The model under review builds one solid part; all positions refer to its coordinate system, in mm. Face numbers are marked on the shaded views. A direction names the side the tool comes from. Coordinates: 2 decimals unless noted, no trailing zeros. Loops run counter-clockwise (first coordinate to the right, second up) from the corner with the lowest first, then second, coordinate; pieces in that order, holes last. Notation, with made-up numbers: M -25.5,-27.75 L 29.5,-27.75 A15 ccw 29.5,-12.75 Z; hole C 61.25,57.5 d5. An arc over 180 degrees is marked long. One line per item, written item: value.
```python
from build123d import *

# Parameters (mm, degrees)
SKETCH1_W           = 10
SKETCH1_H           = 6
BOSS_EXTRUDE1_DEPTH = 3
BOSS_EXTRUDE2_DEPTH = 6
SKETCH3_W           = 0.5
SKETCH3_H           = 2
SKETCH3_W_2         = 1
SKETCH3_H_2         = 3
CUT_EXTRUDE1_DEPTH  = 1.5


with BuildPart() as part:
    # Sketch1 → Boss-Extrude1 (new body)
    with BuildSketch(Plane.XY):
        with Locations((5, 3)):
            Rectangle(SKETCH1_W, SKETCH1_H)
    extrude(amount=BOSS_EXTRUDE1_DEPTH)

    # Sketch2 → Boss-Extrude2 (add)
    with BuildSketch(Plane.XZ):
        Polygon((3.028685262, 4.124905721), (0, 3), (5.333823351, 3), align=None)
        Polygon((7.779518642, 3.625927659), (5.333823351, 3), (10, 3), align=None)
    extrude(amount=-BOSS_EXTRUDE2_DEPTH)

    # Sketch3 → Cut-Extrude1 (cut)
    with BuildSketch(Plane(origin=(0, 0, 0), x_dir=(-1, 0, 0), z_dir=(0, 0, -1))):
        with Locations((-2.75, 3.5)):
            Rectangle(SKETCH3_W, SKETCH3_H)
        with Locations((-6.5, 3)):
            Rectangle(SKETCH3_W_2, SKETCH3_H_2)
    extrude(amount=-CUT_EXTRUDE1_DEPTH, mode=Mode.SUBTRACT)


solid = part.part
```
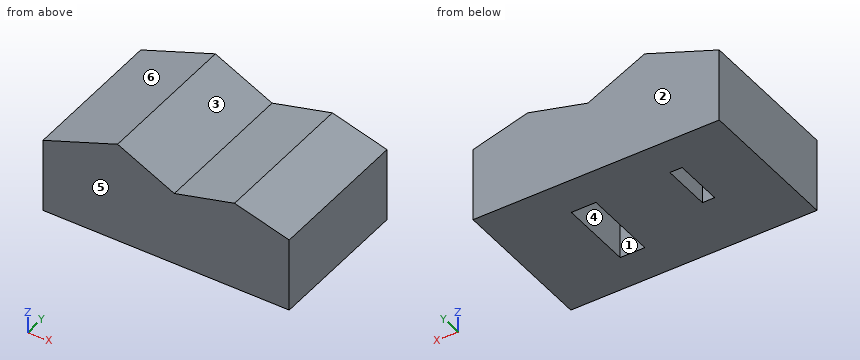
(1) Add section A-A on z = 1.15. State the section outline as (x, y) points.
Checks:
outline: M 0,0 L 10,0 L 10,6 L 0,6 Z; hole M 2.5,2.5 L 3,2.5 L 3,4.5 L 2.5,4.5 Z; hole M 6,1.5 L 7,1.5 L 7,4.5 L 6,4.5 Z
(2) Draft analysis for pull direction X (two halves, no side actions). For the marked faces 4, 5 and 6, state which applies: pulls with the +X half, pulls with the -X half, needs draft (parallel to the pull), parting line crosses it, or undercut.
Checks:
face 4: undercut
face 5: needs draft
face 6: pulls with the -X half
(3) Add section D-D on x = 6.75. State the section outline as (y, z) points, then the cut area to 3 significant figures.
Checks:
outline: M 0,0 L 1.5,0 L 1.5,1.5 L 4.5,1.5 L 4.5,0 L 6,0 L 6,3.36 L 0,3.36 Z
area: 15.7 mm^2
(4) Tool access review of the marked faces 1, 2 and 3: name each direction out of +Z, -Z, +X, -X, +Y, -Y from which nothing blocks a thin tool from reaching the whole face with its end or side.
Checks:
face 1: -Z
face 2: +Z, -Z, +X, -X, +Y
face 3: +Z, +Y, -Y
(5) To check wall thickness, follow L1, parallel to X at y = 3.3, z = 1.05; L2, parallel to Z at x = 9.25, y = 1.2; L3, parallel to Z at x = 2.5, y = 4.8. State the ranges of each line that lie inside material, in increasing order. Write a range as [from, to].
Checks:
L1: [0, 2.5], [3, 6], [7, 10]
L2: [0, 3.21]
L3: [0, 3.93]
(6) Insertion check: pin 1 Ø0.8 at (x, y) = (6.5, 2.5) entering from -Z. The pin has a flat end and moves straight along its axis. Give the tip position at first contact, or say it passes through.
Checks:
pin 1: z = 1.5
(7) Add section B-B on y = 1.75. State the section outline as (x, z) points, then the cut area to 3 significant figures.
Checks:
outline: M 0,0 L 6,0 L 6,1.5 L 7,1.5 L 7,0 L 10,0 L 10,3 L 7.78,3.63 L 5.33,3 L 3.03,4.12 L 0,3 Z
area: 33.0 mm^2
(8) Add section C-C on z = 3.5. State the section outline as (x, y) points.
Checks:
outline: M 1.35,0 L 4.31,0 L 4.31,6 L 1.35,6 Z; M 7.29,0 L 8.23,0 L 8.23,6 L 7.29,6 Z
